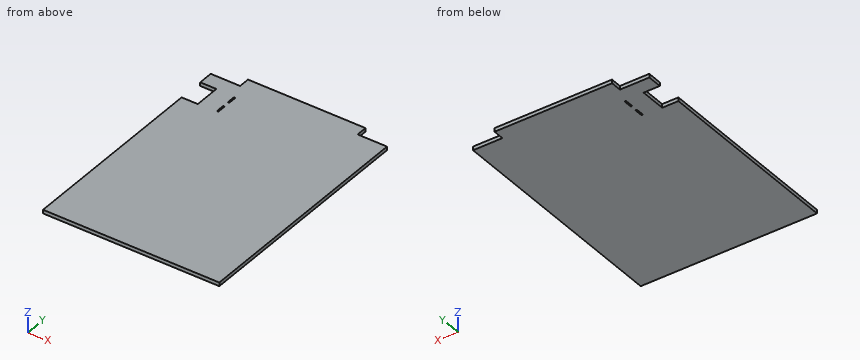
from build123d import *

# Parameters (mm, degrees)
ESQUISSE1_W             = 480
ESQUISSE1_H             = 670
BOSS_EXTRU_1_DEPTH      = 10
ESQUISSE2_W             = 80
ESQUISSE2_H             = 30
ENL_V_MAT_EXTRU_1_DEPTH = 11
ESQUISSE3_W             = 44
ESQUISSE3_H             = 71
ENL_V_MAT_EXTRU_2_DEPTH = 11


with BuildPart() as part:
    # Esquisse1 → Boss.-Extru.1 (new body)
    with BuildSketch(Plane.XY):
        with Locations((-50, 0)):
            Rectangle(ESQUISSE1_W, ESQUISSE1_H)
    extrude(amount=BOSS_EXTRU_1_DEPTH)

    # Esquisse2 → Enlèv. mat.-Extru.1 (cut, through all)
    with BuildSketch(Plane(origin=(0, 0, 0), x_dir=(-1, 0, 0), z_dir=(0, 0, -1))):
        with Locations((-150, 320)):
            Rectangle(ESQUISSE2_W, ESQUISSE2_H)
        with Locations((250, 320)):
            Rectangle(ESQUISSE2_W, ESQUISSE2_H)
    extrude(amount=-ENL_V_MAT_EXTRU_1_DEPTH, mode=Mode.SUBTRACT)

    # Esquisse3 → Enlèv. mat.-Extru.2 (cut, through all)
    with BuildSketch(Plane(origin=(0, 0, 0), x_dir=(-1, 0, 0), z_dir=(0, 0, -1))):
        with BuildLine():
            Line((192, 260), (192, 240))
            ThreePointArc((192, 240), (194, 238), (196, 240))
            Line((196, 240), (196, 260))
            ThreePointArc((196, 260), (194, 262), (192, 260))
        make_face()
        with BuildLine():
            Line((192, 219), (192, 199))
            ThreePointArc((192, 199), (194, 197), (196, 199))
            Line((196, 199), (196, 219))
            ThreePointArc((196, 219), (194, 221), (192, 219))
        make_face()
        with Locations((268, 229.5)):
            Rectangle(ESQUISSE3_W, ESQUISSE3_H)
    extrude(amount=-ENL_V_MAT_EXTRU_2_DEPTH, mode=Mode.SUBTRACT)


solid = part.part
Work out the finished part from the listing and answer in its coordinate system (mm). Give positions to 0.01 mm unless a question says otherwise; leave off trailing zeros. Write each loop counter-clockwise with the first axis right and the second up, starting at its lowest first coordinate (ties: lowest second). Pieces come first, ordered by that corner, then holes. Notation, with made-up numbers: M -8.75,47.25 L 4.25,47.25 A17 ccw 4.25,74.25 Z; hole C 43.25,32.25 d5. An arc over 180 degrees is marked long. Answer as CSV lines item,"result".
Q1. A cutting plane is placed at A-A on z = 8. Write down the section's boundary in (x, y).
A:
outline,"M -290,-335 L 190,-335 L 190,305 L 110,305 L 110,335 L -210,335 L -210,305 L -290,305 L -290,265 L -246,265 L -246,194 L -290,194 Z; hole M -196,199 A2 ccw -192,199 L -192,219 A2 ccw -196,219 Z; hole M -196,240 A2 ccw -192,240 L -192,260 A2 ccw -196,260 Z"
Q2. Find the intervals of material crossed by probe 1 along Y at (x, z) = (-259, 8); probe 2 along X at (y, z) = (235, 1.5); probe 3 along Y at (x, z) = (118.5, 5), in increasing order. Write a range as [from, to].
A:
probe 1,"y = [-335, 194], [265, 305]"
probe 2,"x = [-246, 190]"
probe 3,"y = [-335, 305]"
Q3. A cutting plane is placed at B-B on x = -235.5. Write down the section's boundary in (y, z), plus the area to 3 significant figures.
A:
outline,"M -335,0 L 305,0 L 305,10 L -335,10 Z"
area,"6,400 mm²"
Q4. Given P1, Ø5, axis at x = 147.5, z = 3.5, coming from the +Y side, flat-ended and moving along its own axis, determine where the tip first touches the part or whether it passes through.
A:
P1,"stops at y = 305"
